Design review of the part built by this model. Coordinates are the model's own, in mm. Face numbers are marked on the shaded views. A direction names the side the tool comes from. Give positions to 0.01 mm unless a question says otherwise; leave off trailing zeros. Loops run counter-clockwise (first coordinate to the right, second up) from the corner with the lowest first, then second, coordinate; pieces in that order, holes last. Notation, with made-up numbers: (-27.75, 29.5) - (29.25, 29.5) arc R15 ccw to (29.25, 38.5) - close; hole circle Ø8 at (42, 15.25). An arc over 180 degrees is marked (long way). Write each question's results on one line, items separated by ' | '.
Autodesk Inventor part; units mm, degrees
ref_plane "YZ Plane" through (0, 0, 0) normal (1, 0, 0) x (0, 1, 0)
ref_plane "XZ Plane" through (0, 0, 0) normal (0, 1, 0) x (-1, 0, 0)
ref_plane "XY Plane" through (0, 0, 0) normal (0, 0, 1) x (1, 0, 0)
sketch "Sketch1" plane through (0, 0, 0) normal (0, 1, 0) x (-1, 0, 0)
  line L0 (-9.5, 9.5) -> (9.5, 9.5)
  line L1 (9.5, 9.5) -> (9.5, -9.5)
  line L2 (9.5, -9.5) -> (-9.5, -9.5)
  line L3 (-9.5, -9.5) -> (-9.5, 9.5)
  line L4 (-9.5, 9.5) -> (9.5, -9.5) construction
  line L5 (9.5, 9.5) -> (-9.5, -9.5) construction
  point P0 (0, 0)
extrude "Extrusion1" add sketch "Sketch1" along normal blind 47
sketch "Sketch2" plane through (-9.5, 0, 9.5) normal (0, 0, 1) x (1, 0, 0)
  line L0 (0, 47) -> (19, 47) construction
  line L1 (9.5, 34.5) -> (9.5, 12.5) construction
  line L2 (2.5, 34.5) -> (16.5, 34.5)
  line L3 (16.5, 34.5) -> (16.5, 12.5)
  line L4 (16.5, 12.5) -> (2.5, 12.5)
  line L5 (2.5, 12.5) -> (2.5, 34.5)
  line L6 (2.5, 34.5) -> (16.5, 12.5) construction
  line L7 (16.5, 34.5) -> (2.5, 12.5) construction
  point P0 (9.5, 0)
  point P1 (9.5, 23.5)
  dimension "d5" = 22
  dimension "d6" = 14
  dimension "d7" = 22
extrude "Extrusion2" cut sketch "Sketch2" against normal blind 8
fillet "Fillet1" radius 2 4 edges at (-7, 34.5, 5.5) (-7, 12.5, 5.5) (7, 34.5, 5.5) (7, 12.5, 5.5)
sketch "Sketch3" plane through (0, 47, 0) normal (0, 1, 0) x (1, 0, 0)
  line L0 (9.5, 9.5) -> (-9.5, 9.5) construction
  line L1 (0, 9.5) -> (0, -11.2) construction
  circle A0 centre (0, -11.2) radius 6
  point P0 (0, 0)
  dimension "d11" = 20.7
  dimension "d12" = 12
extrude "Extrusion3" cut sketch "Sketch3" against normal through all
chamfer "Chamfer1" distance 1 angle 45 2 edges at (-9.5, 23.5, -9.5) (9.5, 23.5, -9.5)
properties part number "Semi cuscinetto 2"
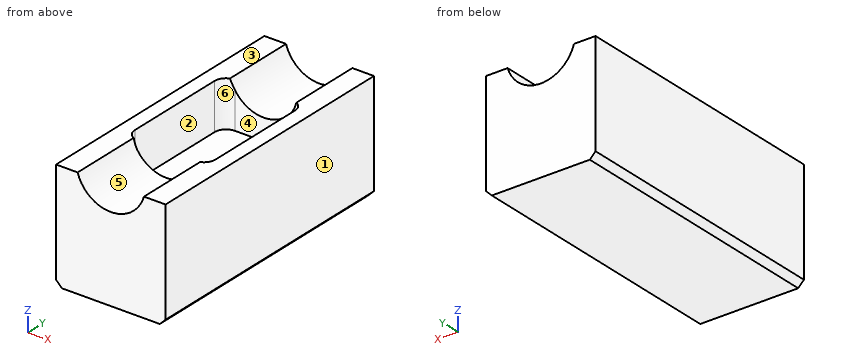
Item 1: Clearance check with a flat-ended pin moving along its axis: P1, Ø7, axis at x = 3, y = 23.5, coming from the +Z side. State where the tip first meets the part, or that it passes through.
Output values:
P1: stops at z = 1.5
Item 2: We need section A-A on z = 4.25. Give the boundary of the cut face in (x, y), then the cut area to 3 significant figures.
Output values:
outline: (-9.5, 0) - (9.5, 0) - (9.5, 47) - (-9.5, 47) - close; hole (-7, 14.5) arc R2 ccw to (-5, 12.5) - (5, 12.5) arc R2 ccw to (7, 14.5) - (7, 32.5) arc R2 ccw to (5, 34.5) - (-5, 34.5) arc R2 ccw to (-7, 32.5) - close | area: 588 mm²
Item 3: We need section D-D on y = 44.5. Give the boundary of the cut face in (x, z).
Output values:
outline: (-9.5, -8.5) - (-8.5, -9.5) - (8.5, -9.5) - (9.5, -8.5) - (9.5, 9.5) - (5.75, 9.5) arc R6 cw to (-5.75, 9.5) - (-9.5, 9.5) - close
Item 4: We need section B-B on y = 20. Give the boundary of the cut face in (x, z), then the cut area to 3 significant figures.
Output values:
outline: (-9.5, -8.5) - (-8.5, -9.5) - (8.5, -9.5) - (9.5, -8.5) - (9.5, 9.5) - (7, 9.5) - (7, 1.5) - (-7, 1.5) - (-7, 9.5) - (-9.5, 9.5) - close | area: 248 mm²
Item 5: Tool access review of the marked faces 5 and 6: name each direction out of +Z, -Z, +X, -X, +Y, -Y from which nothing blocks a thin tool from reaching the whole face with its end or side.
Output values:
face 5: +Z, +Y, -Y | face 6: +Z
Item 6: Wall thickness on probe 1 along Y at (x, z) = (-2.75, 2.5); probe 2 along X at (y, z) = (14.5, 8); probe 3 along Z at (x, y) = (-4.75, 18.5): over which ranges is each line inside the solid? List them lowest first.
Output values:
probe 1: y = 0 to 12.5, 34.5 to 47 | probe 2: x = -9.5 to -7, 7 to 9.5 | probe 3: z = -9.5 to 1.5
Item 7: Draft analysis for pull direction X (two halves, no side actions). For the marked faces 1, 2, 3 and 4, state which applies: +X half, -X half, draft (parallel to the pull), parting line (faces both ways), or undercut.
Output values:
face 1: +X half | face 2: undercut | face 3: draft | face 4: undercut
Item 8: We need section C-C on x = -3.5. Give the boundary of the cut face in (y, z), then the cut area to 3 significant figures.
Output values:
outline: (0, -9.5) - (47, -9.5) - (47, 6.33) - (34.5, 6.33) - (34.5, 1.5) - (12.5, 1.5) - (12.5, 6.33) - (0, 6.33) - close | area: 638 mm²
